```python
from build123d import *

# Parameters (mm, degrees)
SKETCH1_R               = 20
BOSS_EXTRUDE1_DEPTH     = 30
CUT_EXTRUDE1_DEPTH      = 20
SKETCH3_R               = 3
CUT_EXTRUDE2_DEPTH      = 35
CUT_EXTRUDE3_DEPTH      = 28
CUT_EXTRUDE3_DEPTH_BACK = 31
SKETCH4_R               = 6.25
SKETCH5_R               = 2.3
CUT_EXTRUDE4_DEPTH      = 30
SKETCH9_R               = 3.5
BOSS_EXTRUDE4_DEPTH     = 10
CUT_EXTRUDE6_START      = -10
SKETCH11_R              = 3
CUT_EXTRUDE6_DEPTH      = 10


with BuildPart() as part:
    # Sketch1 → Boss-Extrude1 (new body)
    with BuildSketch(Plane.XY):
        Circle(SKETCH1_R)
    extrude(amount=BOSS_EXTRUDE1_DEPTH)

    # Sketch2 → Cut-Extrude1 (cut)
    with BuildSketch(Plane.XY.offset(30)):
        with BuildLine():
            Line((-5, 10), (5, 10))
            ThreePointArc((5, 10), (15, 0), (5, -10))
            Line((5, -10), (-5, -10))
            ThreePointArc((-5, -10), (-15, 0), (-5, 10))
        make_face()
    extrude(amount=-CUT_EXTRUDE1_DEPTH, mode=Mode.SUBTRACT)

    # Sketch3 → Cut-Extrude2 (cut)
    with BuildSketch(Plane.XY.offset(30)):
        with Locations((0, 14.722991755)):
            Circle(SKETCH3_R)
    extrude(amount=-CUT_EXTRUDE2_DEPTH, mode=Mode.SUBTRACT)

    # Sketch4 → Cut-Extrude3 (cut, two sides: drawn at the far end of the back side and taken through both)
    with BuildSketch(Plane(origin=(0, 0, 0), x_dir=(0, 0, -1), z_dir=(1, 0, 0)).offset(-CUT_EXTRUDE3_DEPTH_BACK)):
        with Locations(Location((-19.676237733, 0, 0), (0, 0, 180))):
            Circle(SKETCH4_R)
    extrude(amount=CUT_EXTRUDE3_DEPTH + CUT_EXTRUDE3_DEPTH_BACK, mode=Mode.SUBTRACT)

    # Sketch5 → Cut-Extrude4 (cut)
    with BuildSketch(Plane(origin=(0, 0, 0), x_dir=(-1, 0, 0), z_dir=(0, 0, -1))):
        Circle(SKETCH5_R)
    extrude(amount=-CUT_EXTRUDE4_DEPTH, mode=Mode.SUBTRACT)

    # Sketch9 → Boss-Extrude4 (add)
    with BuildSketch(Plane(origin=(0, 0, 0), x_dir=(-1, 0, 0), z_dir=(0, 0, -1))):
        with Locations(Location((0, 14.722991755, 0), (0, 0, 180))):
            Circle(SKETCH9_R)
    extrude(amount=BOSS_EXTRUDE4_DEPTH)

    # Sketch11 → Cut-Extrude6 (cut)
    with BuildSketch(Plane(origin=(0, 0, -10), x_dir=(-1, 0, 0), z_dir=(0, 0, -1)).offset(CUT_EXTRUDE6_START)):
        with Locations(Location((0, 14.722991755, 0), (0, 0, 180))):
            Circle(SKETCH11_R)
    extrude(amount=CUT_EXTRUDE6_DEPTH, mode=Mode.SUBTRACT)


solid = part.part
```
Read the model definition and answer for the solid it produces. Units are mm, in the model's axes. A direction names the side the tool comes from. Round coordinates to 2 decimals unless told otherwise and drop trailing zeros. Write each loop counter-clockwise with the first axis right and the second up, starting at its lowest first coordinate (ties: lowest second). Pieces come first, ordered by that corner, then holes. Notation, with made-up numbers: (33, -37) - (75, -37) arc R23 cw to (75, -24) - close; hole circle Ø11 at (38.25, 5). An arc over 180 degrees is marked (long way). One line per item, written item: value.
Q1. Find section D-D (x = -16). Determine the outline of the cut face in (y, z).
The answers:
outline: (-12, 0) - (12, 0) - (12, 30) - (-12, 30) - close; hole circle Ø12.5 at (0, 19.68)
Q2. For a pull along Y with two mould halves and no side action, classify faces 4 (the flat face through (-3, 0, 10)), 5 (the cylindrical face through (18.475, -7.66, 14.79)), 6 (the flat face through (0, -4, 0)) as pulls with the +Y half, pulls with the -Y half, needs draft (parallel to the pull), parting line crosses it, or undercut.
The answers:
face 4: undercut
face 5: parting line crosses it
face 6: needs draft
Q3. Find section A-A (y = 0). Determine the outline of the cut face in (x, z).
The answers:
outline: (-20, 0) - (-2.3, 0) - (-2.3, 10) - (-15, 10) - (-15, 13.43) - (-20, 13.43) - close; (-20, 25.93) - (-15, 25.93) - (-15, 30) - (-20, 30) - close; (2.3, 0) - (20, 0) - (20, 13.43) - (15, 13.43) - (15, 10) - (2.3, 10) - close; (15, 25.93) - (20, 25.93) - (20, 30) - (15, 30) - close
Q4. Find section C-C (z = 25). Determine the outline of the cut face in (x, y), and give its area (3 significant figures).
The answers:
outline: (-19.73, -3.27) arc R20 ccw to (19.73, -3.27) - (14.45, -3.27) arc R10 cw to (5, -10) - (-5, -10) arc R10 cw to (-14.45, -3.27) - close; (-19.73, 3.27) - (-14.45, 3.27) arc R10 cw to (-5, 10) - (5, 10) arc R10 cw to (14.45, 3.27) - (19.73, 3.27) arc R20 ccw to start; hole circle Ø6 at (0, 14.72)
area: 648 mm2
Q5. Each of these flat-tipped pins is pushed along its axis until it touches: P1, Ø3, axis at x = -1.5, z = 18, coming from the +Y side; P2, Ø4, axis at y = -7.5, z = 6, coming from the -X side; P3, Ø5, axis at x = 0, y = 14.72, coming from the +Z side; P4, Ø4, axis at x = 10.5, z = 0, coming from the -Y side. Where does it stop, or does it pass through?
The answers:
P1: stops at y = 20
P2: stops at x = -19.23
P3: passes through
P4: stops at y = -18.1
Q6. Find section B-B (x = 0). Determine the outline of the cut face in (y, z), and give its area (3 significant figures).
The answers:
outline: (-20, 0) - (-2.3, 0) - (-2.3, 10) - (-10, 10) - (-10, 30) - (-20, 30) - close; (2.3, 0) - (11.22, 0) - (11.22, -10) - (11.72, -10) - (11.72, 30) - (10, 30) - (10, 10) - (2.3, 10) - close; (17.72, -10) - (18.22, -10) - (18.22, 0) - (20, 0) - (20, 30) - (17.72, 30) - close
area: 584 mm2
Q7. Which of the six approach directions +Z, -Z, +X, -X, +Y, -Y give full straight-line access (tool end or side, diameter ignored) to faces 1 (the flat face through (3, 16, -10)), 2 (the cylindrical face through (1.615, 17.828, -4.93)), 3 (the flat face through (0, 10, 20))?
The answers:
face 1: -Z, +X, -X, +Y, -Y
face 2: -Z
face 3: +Z
Q8. Straight lines are drawn through the part: line 1 (Y direction, x = 0, z = 2); line 2 (Y direction, x = 1, z = 21); line 3 (Z direction, x = 11.5, y = 12). For each, find the intervals that lie inside material, in ascending order. Write a range as from..to.
The answers:
line 1: y = -20..-2.3, 2.3..11.72, 17.72..20
line 2: y = -19.97..-10, 10..11.89, 17.55..19.97
line 3: z = 0..30
